The listing builds one solid part. Answer for the finished solid, in the listing's coordinates (mm). A direction names the side the tool comes from. Coordinates: 2 decimals unless noted, no trailing zeros. Order: outer loops, then holes, each group sorted by start corner. A loop starts at its lowest first (then second) coordinate and runs counter-clockwise, first axis right, second up.
from build123d import *

# Parameters (mm, degrees)
SKETCH1_R            = 76.2
BOSS_EXTRUDE1_DEPTH  = 3.81
SKETCH2_R            = 76.2
SKETCH2_R_2          = 72.39
BOSS_EXTRUDE2_DEPTH  = 12.7
SKETCH3_R            = 4.445
CUT_EXTRUDE1_DEPTH   = 4.81
BOSS_EXTRUDE3_DEPTH  = 12.7
BOSS_EXTRUDE4_DEPTH  = 12.7
BOSS_EXTRUDE5_DEPTH  = 12.7
BOSS_EXTRUDE8_DEPTH  = 12.7
BOSS_EXTRUDE9_DEPTH  = 12.7
BOSS_EXTRUDE10_DEPTH = 12.7
BOSS_EXTRUDE11_DEPTH = 12.7
BOSS_EXTRUDE19_DEPTH = 12.7
BOSS_EXTRUDE20_DEPTH = 12.7
BOSS_EXTRUDE21_DEPTH = 12.7
BOSS_EXTRUDE22_DEPTH = 12.7


with BuildPart() as part:
    # Sketch1 → Boss-Extrude1 (new body)
    with BuildSketch(Plane(origin=(0, 0, 0), x_dir=(1, 0, 0), z_dir=(0, 1, 0))):
        Circle(SKETCH1_R)
    extrude(amount=BOSS_EXTRUDE1_DEPTH)

    # Sketch2 → Boss-Extrude2 (add)
    with BuildSketch(Plane(origin=(0, 3.81, 0), x_dir=(1, 0, 0), z_dir=(0, 1, 0))):
        Circle(SKETCH2_R)
        Circle(SKETCH2_R_2, mode=Mode.SUBTRACT)
    extrude(amount=BOSS_EXTRUDE2_DEPTH)

    # Sketch3 → Cut-Extrude1 (cut, through all)
    with BuildSketch(Plane(origin=(0, 3.81, 0), x_dir=(1, 0, 0), z_dir=(0, 1, 0))):
        Circle(SKETCH3_R)
    extrude(amount=-CUT_EXTRUDE1_DEPTH, mode=Mode.SUBTRACT)

    # Sketch4 → Boss-Extrude3 (add)
    with BuildSketch(Plane(origin=(0, 3.81, 0), x_dir=(1, 0, 0), z_dir=(0, 1, 0))):
        with BuildLine():
            Line((0, 7.62), (0, 10.16))
            ThreePointArc((0, 10.16), (-10.16, 0), (0, -10.16))
            Line((0, -10.16), (0, -7.62))
            ThreePointArc((0, -7.62), (-7.62, 0), (0, 7.62))
        make_face()
    extrude(amount=BOSS_EXTRUDE3_DEPTH)

    # Sketch5 → Boss-Extrude4 (add)
    with BuildSketch(Plane(origin=(0, 3.81, 0), x_dir=(1, 0, 0), z_dir=(0, 1, 0))):
        Polygon((0, -10.16), (0, -25.176651115), (-2.54, -25.176651115), (-2.520078124, -9.8425), align=None)
    extrude(amount=BOSS_EXTRUDE4_DEPTH)

    # Sketch6 → Boss-Extrude5 (add)
    with BuildSketch(Plane(origin=(0, 3.81, 0), x_dir=(1, 0, 0), z_dir=(0, 1, 0))):
        with BuildLine():
            Line((-21.983467268, -12.265166189), (-24.2679054, -13.539715513))
            ThreePointArc((-24.2679054, -13.539715513), (17.868925405, 21.282777862), (-9.135212339, -26.245057138))
            Line((-9.135212339, -26.245057138), (-8.472154438, -23.705057138))
            ThreePointArc((-8.472154438, -23.705057138), (16.266652993, 19.212057025), (-21.983467268, -12.265166189))
        make_face()
    extrude(amount=BOSS_EXTRUDE5_DEPTH)

    # Sketch7 → Boss-Extrude8 (add)
    with BuildSketch(Plane(origin=(0, 3.81, 0), x_dir=(1, 0, 0), z_dir=(0, 1, 0))):
        Polygon((9.247520886, -26.205695681), (15.12853456, -40.45434823), (17.476408475, -39.485282661), (11.601678734, -25.251854966), align=None)
    extrude(amount=BOSS_EXTRUDE8_DEPTH)

    # Sketch8 → Boss-Extrude9 (add)
    with BuildSketch(Plane(origin=(0, 3.81, 0), x_dir=(1, 0, 0), z_dir=(0, 1, 0))):
        with BuildLine():
            Line((-0.983739015, -43.049055689), (-0.983739015, -45.589055689))
            ThreePointArc((-0.983739015, -45.589055689), (18.37519714, -41.733462247), (34.290907527, -30.05766794))
            Line((34.290907527, -30.05766794), (32.345154642, -28.424987411))
            ThreePointArc((32.345154642, -28.424987411), (17.301746755, -39.431440468), (-0.983739015, -43.049055689))
        make_face()
    extrude(amount=BOSS_EXTRUDE9_DEPTH)

    # Sketch9 → Boss-Extrude10 (add)
    with BuildSketch(Plane(origin=(0, 3.81, 0), x_dir=(1, 0, 0), z_dir=(0, 1, 0))):
        Polygon((-9.684496714, 26.047373228), (-12.022324897, 25.054317646), (-17.646368783, 39.218629503), (-15.3085406, 40.211685084), align=None)
    extrude(amount=BOSS_EXTRUDE10_DEPTH)

    # Sketch10 → Boss-Extrude11 (add)
    with BuildSketch(Plane(origin=(0, 3.81, 0), x_dir=(1, 0, 0), z_dir=(0, 1, 0))):
        with BuildLine():
            Line((0, 43.18), (0, 45.72))
            ThreePointArc((0, 45.72), (-19.322106927, 41.436392023), (-35.023551939, 29.388249515))
            Line((-35.023551939, 29.388249515), (-33.077799054, 27.755568986))
            ThreePointArc((-33.077799054, 27.755568986), (-18.248656542, 39.134370244), (0, 43.18))
        make_face()
    extrude(amount=BOSS_EXTRUDE11_DEPTH)

    # Sketch15 → Boss-Extrude19 (add)
    with BuildSketch(Plane(origin=(0, 16.51, 0), x_dir=(1, 0, 0), z_dir=(0, 1, 0))):
        with BuildLine():
            Line((18.813236265, 54.331808343), (17.982135906, 51.931626642))
            ThreePointArc((17.982135906, 51.931626642), (49.436495597, 24.005915117), (51.931626642, -17.982135906))
            Line((51.931626642, -17.982135906), (54.331808343, -18.813236265))
            ThreePointArc((54.331808343, -18.813236265), (51.721357052, 25.115423174), (18.813236265, 54.331808343))
        make_face()
    extrude(amount=-BOSS_EXTRUDE19_DEPTH)

    # Sketch16 → Boss-Extrude20 (add)
    with BuildSketch(Plane(origin=(0, 3.81, 0), x_dir=(1, 0, 0), z_dir=(0, 1, 0))):
        Polygon((62.923710936, 35.479950277), (64.179700672, 33.272216194), (50.933296173, 25.736277775), (49.677306437, 27.944011858), align=None)
    extrude(amount=BOSS_EXTRUDE20_DEPTH)

    # Sketch17 → Boss-Extrude21 (add)
    with BuildSketch(Plane(origin=(0, 3.81, 0), x_dir=(1, 0, 0), z_dir=(0, 1, 0))):
        Polygon((-69.78543957, -19.725953422), (-68.982438616, -22.135681513), (-54.524070075, -17.317675793), (-55.327071028, -14.907947702), align=None)
    extrude(amount=BOSS_EXTRUDE21_DEPTH)

    # Sketch18 → Boss-Extrude22 (add)
    with BuildSketch(Plane(origin=(0, 3.81, 0), x_dir=(1, 0, 0), z_dir=(0, 1, 0))):
        with BuildLine():
            Line((-24.16501099, -51.873510961), (-23.092435835, -49.571081258))
            ThreePointArc((-23.092435835, -49.571081258), (-49.553841631, -23.129407029), (-52.827537989, 14.135201447))
            Line((-52.827537989, 14.135201447), (-55.281645892, 14.790149527))
            ThreePointArc((-55.281645892, 14.790149527), (-51.855122504, -24.204445165), (-24.16501099, -51.873510961))
        make_face()
    extrude(amount=BOSS_EXTRUDE22_DEPTH)


solid = part.part
1) Determine the mould class of faces 3 (the face through (-10.053, 10.071, -1.474)), 4 (the face through (16, 0, -1)) for opening direction Z: released by +Z, released by -Z, zero draft, split by the parting line, or undercut.
2) A tool of negligible diameter and unlimited length cuts with its end or side. For faces 1 (the face through (14.557, 10.071, 32.412)), 2 (the face through (50, 16.51, -26)), from which of +Z, -Z, +X, -X, +Y, -Y can it reach the whole face along a straight path? Write none if from no direction.
3) Consider L1, parallel to Z at x = 0, y = 1.55 (3 decimals); L2, parallel to Z at x = -37, y = 10.75. Determine where each line is inside the solid, lowest interval first.
4) Section A-A (y = 8.75) is taken. Give the number of separate pieces and of enclosed holes in the cut face, then the cut area to 3 significant figures.
5) Section B-B (z = -64.5) is taken. Give the vertices of the cut face in (x, y).
6) Each of these flat-tipped pins is pushed along its axis until it touches: P1, Ø1.5, axis at x = 33.5, z = 25.5, coming from the +Y side; P2, Ø2, axis at x = 32, y = 10.5, coming from the +Z side; P3, Ø0.8, axis at y = 13, z = 44, coming from the -X side; P4, Ø8, axis at x = 23, z = -10, coming from the +Y side. Where does it stop, or does it pass through?
Filled sheet:
1. face 3: undercut
1. face 4: zero draft
2. face 1: +Y
2. face 2: +Z, -Z, +X, -X, +Y
3. L1: z = -76.2 to -4.445, 4.445 to 76.2
3. L2: z = -66.61 to -62.22, 40.27 to 43.66, 62.22 to 66.61
4. separate pieces: 4
4. enclosed holes: 1
4. area: 3,050 mm2
5. outline: (-40.57, 0) - (40.57, 0) - (40.57, 16.51) - (32.86, 16.51) - (32.86, 3.81) - (-32.86, 3.81) - (-32.86, 16.51) - (-40.57, 16.51) - close
6. P1: stops at y = 3.81
6. P2: stops at z = 69.61
6. P3: stops at x = -62.49
6. P4: stops at y = 16.51
